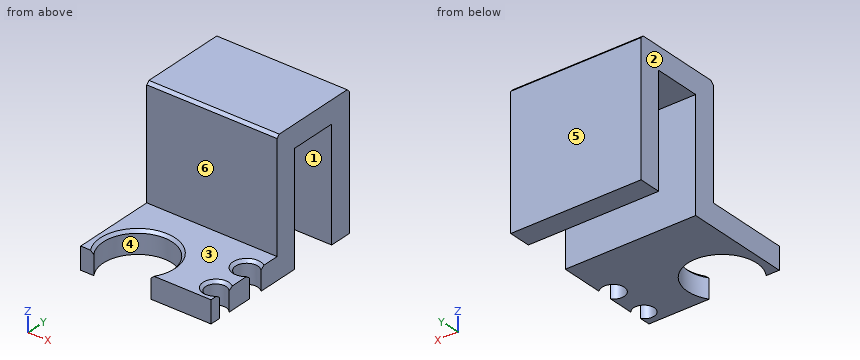
```python
from build123d import *

# Parameters (mm, degrees)
BOX_W             = 31
BOX_H             = 8.4
BOX_DEPTH         = 20
CYLINDER_R        = 6.225
CYLINDER_DEPTH    = 10
CYLINDER001_R     = 2
CYLINDER001_DEPTH = 10
CYLINDER002_R     = 1.85
CYLINDER002_DEPTH = 10
BOX003_W          = 23.5
BOX003_H          = 4
BOX003_DEPTH      = 24
BOX002_W          = 23.5
BOX002_H          = 16
BOX002_DEPTH      = 4
BOX001_W          = 23.5
BOX001_H          = 4
BOX001_DEPTH      = 24
BOX004_W          = 23.5
BOX004_H          = 14
BOX004_DEPTH      = 4
CHAMFER_SIZE      = 0.5
CHAMFER001_SIZE   = 0.5


with BuildPart() as glass:
    # Box → Box (new body)
    with BuildSketch(Plane(origin=(-10, 0, 0), x_dir=(1, 0, 0), z_dir=(0, 0, 1))):
        with Locations((15.5, 4.2)):
            Rectangle(BOX_W, BOX_H)
    extrude(amount=BOX_DEPTH)


with BuildPart() as obj1:
    # Cylinder → Cylinder (new body)
    with BuildSketch(Plane(origin=(-2.5, -15.5, 0), x_dir=(1, 0, 0), z_dir=(0, 0, 1))):
        Circle(CYLINDER_R)
    extrude(amount=CYLINDER_DEPTH)


with BuildPart() as temp_tube:
    # Cylinder001 → Cylinder001 (new body)
    with BuildSketch(Plane(origin=(12, -9, 0), x_dir=(1, 0, 0), z_dir=(0, 0, 1))):
        Circle(CYLINDER001_R)
    extrude(amount=CYLINDER001_DEPTH)


with BuildPart() as obj2:
    # Cylinder002 → Cylinder002 (new body)
    with BuildSketch(Plane(origin=(12, -16, 0), x_dir=(1, 0, 0), z_dir=(0, 0, 1))):
        Circle(CYLINDER002_R)
    extrude(amount=CYLINDER002_DEPTH)


with BuildPart() as back:
    # Box003 → Box003 (new body)
    with BuildSketch(Plane(origin=(-10, 8.4, 0), x_dir=(1, 0, 0), z_dir=(0, 0, 1))):
        with Locations((11.75, 2)):
            Rectangle(BOX003_W, BOX003_H)
    extrude(amount=BOX003_DEPTH)


with BuildPart() as bottom:
    # Box002 → Box002 (new body)
    with BuildSketch(Plane(origin=(-10, -19, 0), x_dir=(1, 0, 0), z_dir=(0, 0, 1))):
        with Locations((11.75, 8)):
            Rectangle(BOX002_W, BOX002_H)
    extrude(amount=BOX002_DEPTH)


with BuildPart() as front:
    # Box001 → Box001 (new body)
    with BuildSketch(Plane(origin=(-10, -4, 0), x_dir=(1, 0, 0), z_dir=(0, 0, 1))):
        with Locations((11.75, 2)):
            Rectangle(BOX001_W, BOX001_H)
    extrude(amount=BOX001_DEPTH)


with BuildPart() as chamfer001:
    # Box004 → Box004 (new body)
    with BuildSketch(Plane(origin=(-10, -4, 20), x_dir=(1, 0, 0), z_dir=(0, 0, 1))):
        with Locations((11.75, 7)):
            Rectangle(BOX004_W, BOX004_H)
    extrude(amount=BOX004_DEPTH)

    # Fusion: union Back, Bottom, Front
    add(back.part)
    add(bottom.part)
    add(front.part)

    # Cut: cut obj2
    add(obj2.part, mode=Mode.SUBTRACT)

    # Cut001: cut Temp_tube
    add(temp_tube.part, mode=Mode.SUBTRACT)

    # Cut002: cut obj1
    add(obj1.part, mode=Mode.SUBTRACT)

    # Cut003: cut Glass
    add(glass.part, mode=Mode.SUBTRACT)

    # Chamfer
    chamfer_edges = [chamfer001.edges().sort_by_distance(p)[0] for p in [
        (10, -9, 4),
        (10.15, -16, 4),
        (3.449628, -17.330997, 4),
        (-4.330997, -9.550372, 4),
    ]]
    chamfer(chamfer_edges, length=CHAMFER_SIZE)

    # Chamfer001
    chamfer001_edges = [chamfer001.edges().sort_by_distance(p)[0] for p in [
        (1.75, -4, 24),
        (1.75, 12.4, 24),
    ]]
    chamfer(chamfer001_edges, length=CHAMFER001_SIZE)


solid = chamfer001.part
```
CAD build for the part. Positions are in the model's coordinates, mm. Face numbers are marked on the shaded views. A direction names the side the tool comes from. Coordinates: 2 decimals unless noted, no trailing zeros. Write each loop counter-clockwise with the first axis right and the second up, starting at its lowest first coordinate (ties: lowest second). Pieces come first, ordered by that corner, then holes. Notation, with made-up numbers: (58, 75.5) -> (81, 75.5) arc R11 ccw to (81, 88.5) -> close; hole circle Ø5 at (40, 40.25). An arc over 180 degrees is marked (long way). Return JSON: item names as keys, results as strings. Group by question number.
Q1. Cut at D-D, the plane y = -5. Give the cut face in (x, z).
Q2. Which spindle directions (+Z, -Z, +X, -X, +Y, -Y) get a long thin tool onto all of the face, cutting with end or side? Do the marked faces 1, 2 and 3. Say none if no direction does.
Q3. Cut at B-B, the plane z = 5. Give the cut face in (x, y).
Q4. Pull direction Y, two halves, no side cores. Call the marked faces 4, 5 and 6: released by +Y, released by -Y, zero draft, split by the parting line, or undercut.
Q5. Flat gauge pins, fed straight in: pin 1 (10 mm diameter, centred on x = 4.5, z = 14, fed in from -Y); pin 2 (6 mm diameter, centred on x = -7, y = -9, fed in from +Z); pin 3 (10 mm diameter, centred on x = -1.5, z = 7.5, fed in from -Y). Where does each tip first touch, or does it go through?
Q6. Cut at A-A, the plane x = 12. Give the cut face in (y, z).
Q7. Drill centre lines: line 1 (Y direction, x = 12, z = 1.45); line 2 (Y direction, x = 12.75, z = 7); line 3 (Y direction, x = -2.5, z = 0.8) (3 decimals). Where is each one in solid material? Low to high.
Q8. Cut at C-C, the plane x = -2.5. Give the cut face in (y, z) (3 decimals).
Returned:
{
 "1": {"outline": "(-10, 0) -> (13.5, 0) -> (13.5, 4) -> (-10, 4) -> close"},
 "2": {"face 1": "-Z, +X, -X", "face 2": "+Z, -Z, -X, +Y, -Y", "face 3": "+Z, +X, -X, -Y"},
 "3": {"outline": "(-10, -4) -> (13.5, -4) -> (13.5, 0) -> (-10, 0) -> close; (-10, 8.4) -> (13.5, 8.4) -> (13.5, 12.4) -> (-10, 12.4) -> close"},
 "4": {"face 4": "undercut", "face 5": "released by +Y", "face 6": "released by -Y"},
 "5": {"pin 1": "stops at y = -4", "pin 2": "stops at z = 4", "pin 3": "stops at y = -10.73"},
 "6": {"outline": "(-19, 0) -> (-17.85, 0) -> (-17.85, 3.5) -> (-18.35, 4) -> (-19, 4) -> close; (-14.15, 0) -> (-11, 0) -> (-11, 3.5) -> (-11.5, 4) -> (-13.65, 4) -> (-14.15, 3.5) -> close; (-7, 0) -> (0, 0) -> (0, 20) -> (8.4, 20) -> (8.4, 0) -> (12.4, 0) -> (12.4, 23.5) -> (11.9, 24) -> (-3.5, 24) -> (-4, 23.5) -> (-4, 4) -> (-6.5, 4) -> (-7, 3.5) -> close"},
 "7": {"line 1": "y = -19 to -17.85, -14.15 to -11, -7 to 0, 8.4 to 12.4", "line 2": "y = -4 to 0, 8.4 to 12.4", "line 3": "y = -9.275 to 0, 8.4 to 12.4"},
 "8": {"outline": "(-9.275, 0) -> (0, 0) -> (0, 20) -> (8.4, 20) -> (8.4, 0) -> (12.4, 0) -> (12.4, 23.5) -> (11.9, 24) -> (-3.5, 24) -> (-4, 23.5) -> (-4, 4) -> (-8.775, 4) -> (-9.275, 3.5) -> close"}
}
